Model file for the job. Use its own axes, mm. A direction names the side the tool comes from. Give positions to 0.01 mm unless a question says otherwise; leave off trailing zeros. Write each loop counter-clockwise with the first axis right and the second up, starting at its lowest first coordinate (ties: lowest second). Pieces come first, ordered by that corner, then holes. Notation, with made-up numbers: (83.5, 75) - (119.5, 75) arc R15 ccw to (119.5, 95) - close; hole circle Ø5 at (74.25, -37.75). An arc over 180 degrees is marked (long way). Use CSV: the item, a comma, the result in double quotes.
from build123d import *

# Parameters (mm, degrees)
EXTRUDE_1_DEPTH     = 28
EXTRUDE_START       = 28
EXTRUDE_2_DEPTH     = 3
EXTRUDE_3_DEPTH     = 1.5
EXTRUDE_START_2     = -28
EXTRUDE_4_DEPTH     = 3
CUT_EXTRUDE_1_REACH = 47.651
SKETCH_3_R          = 2.2
CUT_EXTRUDE_2_REACH = 47.651
SKETCH_4_R          = 1.7


with BuildPart() as part:
    # 草图1 → 凸台-拉伸1 (new, symmetric)
    with BuildSketch(Plane.XY):
        Polygon((0, 0), (0, 20), (30, 20), (30, 17), (3, 17), (3, 0), align=None)
    extrude(amount=EXTRUDE_1_DEPTH, both=True)

    # 草图2 → 凸台-拉伸2 (add)
    with BuildSketch(Plane.XY.offset(EXTRUDE_START)):
        Polygon((3, 0), (5, 0), (30, 15), (30, 17), (3, 17), align=None)
    extrude(amount=-EXTRUDE_2_DEPTH)

    # 草图2<2> → 凸台-拉伸3 (add, symmetric)
    with BuildSketch(Plane.XY):
        Polygon((3, 0), (5, 0), (30, 15), (30, 17), (3, 17), align=None)
    extrude(amount=EXTRUDE_3_DEPTH, both=True)

    # 草图2<3> → 凸台-拉伸4 (add)
    with BuildSketch(Plane.XY.offset(EXTRUDE_START_2)):
        Polygon((3, 0), (5, 0), (30, 15), (30, 17), (3, 17), align=None)
    extrude(amount=EXTRUDE_4_DEPTH)

    # 草图3 → 切除-拉伸1 (cut, up to next)
    with BuildSketch(Plane(origin=(0, 0, 0), x_dir=(1, 0, 0), z_dir=(0, 1, 0)), mode=Mode.PRIVATE) as cut_extrude_1_sk1:
        with Locations(Location((18.8, 18, 0), (0, 0, 90))):
            Circle(SKETCH_3_R)
    cut_extrude_1_tool1 = extrude(cut_extrude_1_sk1.sketch, amount=CUT_EXTRUDE_1_REACH, mode=Mode.PRIVATE) & part.part
    # 草图3 → 切除-拉伸1 (cut, up to next)
    with BuildSketch(Plane(origin=(0, 0, 0), x_dir=(1, 0, 0), z_dir=(0, 1, 0)), mode=Mode.PRIVATE) as cut_extrude_1_sk2:
        with Locations(Location((18.8, -18, 0), (0, 0, 90))):
            Circle(SKETCH_3_R)
    cut_extrude_1_tool2 = extrude(cut_extrude_1_sk2.sketch, amount=CUT_EXTRUDE_1_REACH, mode=Mode.PRIVATE) & part.part
    add(cut_extrude_1_tool1.solids().sort_by_distance((18.8, 0, -18))[0], mode=Mode.SUBTRACT)
    add(cut_extrude_1_tool2.solids().sort_by_distance((18.8, 0, 18))[0], mode=Mode.SUBTRACT)

    # 草图4 → 切除-拉伸2 (cut, up to next)
    with BuildSketch(Plane(origin=(0, 0, 0), x_dir=(0, 0, -1), z_dir=(1, 0, 0)), mode=Mode.PRIVATE) as cut_extrude_2_sk1:
        with Locations(Location((-18, 10, 0), (0, 0, 180))):
            Circle(SKETCH_4_R)
    cut_extrude_2_tool1 = extrude(cut_extrude_2_sk1.sketch, amount=CUT_EXTRUDE_2_REACH, mode=Mode.PRIVATE) & part.part
    # 草图4 → 切除-拉伸2 (cut, up to next)
    with BuildSketch(Plane(origin=(0, 0, 0), x_dir=(0, 0, -1), z_dir=(1, 0, 0)), mode=Mode.PRIVATE) as cut_extrude_2_sk2:
        with Locations(Location((18, 10, 0), (0, 0, 180))):
            Circle(SKETCH_4_R)
    cut_extrude_2_tool2 = extrude(cut_extrude_2_sk2.sketch, amount=CUT_EXTRUDE_2_REACH, mode=Mode.PRIVATE) & part.part
    add(cut_extrude_2_tool1.solids().sort_by_distance((0, 10, 18))[0], mode=Mode.SUBTRACT)
    add(cut_extrude_2_tool2.solids().sort_by_distance((0, 10, -18))[0], mode=Mode.SUBTRACT)


solid = part.part
(1) 3-axis set-ups, long thin cutter, end or side, ignore diameter. For faces 4 (the face through (17, 17, -13)), 5 (the face through (19.643, 18.479, 15.968)): which of +Z, -Z, +X, -X, +Y, -Y reach the whole face in a straight line?
Checked values:
face 4,"+X, -Y"
face 5,"+Y, -Y"
(2) Saw through at D-D, the plane y = 10. List the corners of the cut face in (x, z).
Checked values:
outline,"(0, -28) - (21.67, -28) - (21.67, -25) - (3, -25) - (3, -19.7) - (0, -19.7) - close; (0, -16.3) - (3, -16.3) - (3, -1.5) - (21.67, -1.5) - (21.67, 1.5) - (3, 1.5) - (3, 16.3) - (0, 16.3) - close; (0, 19.7) - (3, 19.7) - (3, 25) - (21.67, 25) - (21.67, 28) - (0, 28) - close"
(3) Pull direction Z, two halves, no side cores. Call faces 1 (the face through (17.33, 7.4, 26.52)), 2 (the face through (11, 12, 28)), 3 (the face through (13, 11, 25)): released by +Z, released by -Z, zero draft, split by the parting line, or undercut.
Checked values:
face 1,"zero draft"
face 2,"released by +Z"
face 3,"undercut"
(4) Flat gauge pins, fed straight in: P1, Ø5, axis at y = 8, z = -11, coming from the +X side; P2, Ø12, axis at x = 10.5, z = -9.5, coming from the -Y side. Where does each tip first touch, or does it go through?
Checked values:
P1,"stops at x = 3"
P2,"stops at y = 17"
(5) Saw through at B-B, the plane x = 18.8. List the corners of the cut face in (y, z), then the cut area to 3 significant figures.
Checked values:
outline,"(8.28, -28) - (20, -28) - (20, -20.2) - (17, -20.2) - (17, -25) - (8.28, -25) - close; (8.28, -1.5) - (17, -1.5) - (17, -15.8) - (20, -15.8) - (20, 15.8) - (17, 15.8) - (17, 1.5) - (8.28, 1.5) - close; (8.28, 25) - (17, 25) - (17, 20.2) - (20, 20.2) - (20, 28) - (8.28, 28) - close"
area,"220 mm^2"
(6) Wall check: probe 1 along Z at (x, y) = (16, 10.5); probe 2 along Z at (x, y) = (0.8, 10); probe 3 along X at (y, z) = (13.25, -15). Give the ranges that are in metal, low to high. Write a range as [from, to].
Checked values:
probe 1,"z = [-28, -25], [-1.5, 1.5], [25, 28]"
probe 2,"z = [-28, -19.7], [-16.3, 16.3], [19.7, 28]"
probe 3,"x = [0, 3]"
(7) Saw through at C-C, the plane x = 7.25. List the corners of the cut face in (y, z), then the cut area to 3 significant figures.
Checked values:
outline,"(1.35, -28) - (20, -28) - (20, 28) - (1.35, 28) - (1.35, 25) - (17, 25) - (17, 1.5) - (1.35, 1.5) - (1.35, -1.5) - (17, -1.5) - (17, -25) - (1.35, -25) - close"
area,"309 mm^2"
(8) Saw through at A-A, the plane z = 18. List the corners of the cut face in (x, y).
Checked values:
outline,"(0, 0) - (3, 0) - (3, 8.3) - (0, 8.3) - close; (0, 11.7) - (3, 11.7) - (3, 17) - (16.6, 17) - (16.6, 20) - (0, 20) - close; (21, 17) - (30, 17) - (30, 20) - (21, 20) - close"
